Build history of the part. All positions in model axes, mm. Face numbers are marked on the shaded views. A direction names the side the tool comes from. Give positions to 0.01 mm unless a question says otherwise; leave off trailing zeros. Order: outer loops, then holes, each group sorted by start corner. A loop starts at its lowest first (then second) coordinate and runs counter-clockwise, first axis right, second up. Notation, with made-up numbers: M -17,23.25 L 1,23.25 A12 cw 1,33.25 Z; hole C 76.25,-29 d7. An arc over 180 degrees is marked long. Use CSV: the item, a comma, the result in double quotes. Start each with the question number.
Item 1: Band-saw the part on C-C on y = 7. Write the cut outline in (x, z).
Item 2: Two-plate mould, pull along X, no slides. Class the marked faces 3, 4 and 5: pulls with the +X half, pulls with the -X half, needs draft (parallel to the pull), parting line crosses it, or undercut.
Item 3: Pin check, flat tips, straight feed: P1, Ø1, axis at x = -8, y = 8, coming from the +Z side; P2, Ø7.5, axis at x = 2, z = 32.5, coming from the +Y side; P3, Ø0.9, axis at x = 3.5, z = -1, coming from the -Y side. Stop position of each tip, or through.
Item 4: Band-saw the part on A-A on z = 18.5. Write the cut outline in (x, y).
Item 5: Band-saw the part on B-B on x = 8.5. Write the cut outline in (y, z).
Item 6: Wall check: line 1 along Y through (x, z) = (1.5, 18.5); line 2 along X through (y, z) = (3.75, 29); line 3 along Z through (x, y) = (-9.5, -8). Give the ranges that are in metal, low to high.
Item 7: Which spindle directions (+Z, -Z, +X, -X, +Y, -Y) get a long thin tool onto all of the face, cutting with end or side? Do the marked faces 1 and 2. Say none if no direction does.
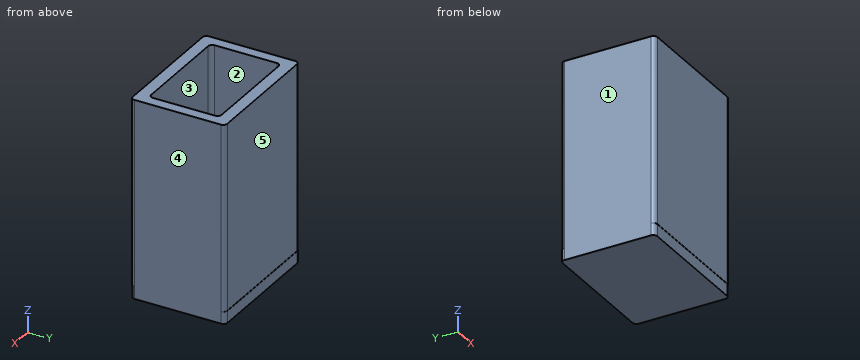
from build123d import *

# Parameters (mm, degrees)
BOSS_EXTRUDE1_DEPTH = 46.3
BOSS_EXTRUDE2_DEPTH = 3


with BuildPart() as part:
    # Sketch1 → Boss-Extrude1 (new body)
    with BuildSketch(Plane.XY):
        with BuildLine():
            Line((-15, 11.75), (15, 11.75))
            ThreePointArc((15, 11.75), (15.707106781, 11.457106781), (16, 10.75))
            Line((16, 10.75), (16, -10.75))
            ThreePointArc((16, -10.75), (15.707106781, -11.457106781), (15, -11.75))
            Line((15, -11.75), (-15, -11.75))
            ThreePointArc((-15, -11.75), (-15.707106781, -11.457106781), (-16, -10.75))
            Line((-16, -10.75), (-16, 10.75))
            ThreePointArc((-16, 10.75), (-15.707106781, 11.457106781), (-15, 11.75))
        make_face()
        with BuildLine():
            Line((-12.25, 8.75), (12.25, 8.75))
            ThreePointArc((12.25, 8.75), (12.957106781, 8.457106781), (13.25, 7.75))
            Line((13.25, 7.75), (13.25, -7.75))
            ThreePointArc((13.25, -7.75), (12.957106781, -8.457106781), (12.25, -8.75))
            Line((12.25, -8.75), (-12.25, -8.75))
            ThreePointArc((-12.25, -8.75), (-12.957106781, -8.457106781), (-13.25, -7.75))
            Line((-13.25, -7.75), (-13.25, 7.75))
            ThreePointArc((-13.25, 7.75), (-12.957106781, 8.457106781), (-12.25, 8.75))
        make_face(mode=Mode.SUBTRACT)
    extrude(amount=BOSS_EXTRUDE1_DEPTH)

    # Sketch3 → Boss-Extrude2 (add)
    with BuildSketch(Plane.XY):
        with BuildLine():
            Line((-15, 11.8), (15, 11.8))
            ThreePointArc((15, 11.8), (15.707106781, 11.507106781), (16, 10.8))
            Line((16, 10.8), (16, -10.7))
            ThreePointArc((16, -10.7), (15.707106781, -11.407106781), (15, -11.7))
            Line((15, -11.7), (-15, -11.7))
            ThreePointArc((-15, -11.7), (-15.707106781, -11.407106781), (-16, -10.7))
            Line((-16, -10.7), (-16, 10.8))
            ThreePointArc((-16, 10.8), (-15.707106781, 11.507106781), (-15, 11.8))
        make_face()
    extrude(amount=-BOSS_EXTRUDE2_DEPTH)


solid = part.part
Model answer:
1,outline,"M -16,-3 L 16,-3 L 16,46.3 L 13.25,46.3 L 13.25,0 L -13.25,0 L -13.25,46.3 L -16,46.3 Z"
2,face 3,"undercut"
2,face 4,"pulls with the +X half"
2,face 5,"needs draft"
3,P1,"stops at z = 0"
3,P2,"stops at y = 11.75"
3,P3,"stops at y = -11.7"
4,outline,"M -16,-10.75 A1 ccw -15,-11.75 L 15,-11.75 A1 ccw 16,-10.75 L 16,10.75 A1 ccw 15,11.75 L -15,11.75 A1 ccw -16,10.75 Z; hole M -13.25,-7.75 A1 ccw -12.25,-8.75 L 12.25,-8.75 A1 ccw 13.25,-7.75 L 13.25,7.75 A1 ccw 12.25,8.75 L -12.25,8.75 A1 ccw -13.25,7.75 Z"
5,outline,"M -11.75,0 L -11.7,0 L -11.7,-3 L 11.8,-3 L 11.8,0 L 11.75,0 L 11.75,46.3 L 8.75,46.3 L 8.75,0 L -8.75,0 L -8.75,46.3 L -11.75,46.3 Z"
6,line 1,"y = -11.75 to -8.75, 8.75 to 11.75"
6,line 2,"x = -16 to -13.25, 13.25 to 16"
6,line 3,"z = -3 to 0"
7,face 1,"+Z, -Z, -X, +Y, -Y"
7,face 2,"+Z"
